from build123d import *

# Parameters (mm, degrees)
SKETCH1_W                 = 127
SKETCH1_H                 = 127
BOSS_EXTRUDE1_DEPTH       = 3.175
SKETCH2_W                 = 3.175
SKETCH2_H                 = 25.4
CUT_EXTRUDE1_DEPTH        = 6.35
LPATTERN1_COUNT           = 3
LPATTERN1_PITCH           = 50.8
LPATTERN1_COUNT_DIR2      = 2
LPATTERN1_PITCH_DIR2      = 123.825
SKETCH3_W                 = 25.4
SKETCH3_H                 = 3.175
CUT_EXTRUDE2_DEPTH        = 6.35
LPATTERN2_COUNT           = 3
LPATTERN2_PITCH           = 50.8
LPATTERN2_COUNT_DIR2      = 2
LPATTERN2_PITCH_DIR2      = 123.825
SKETCH4_W                 = 17.145
SKETCH4_H                 = 4.3942
SKETCH4_W_2               = 3.302
SKETCH4_H_2               = 8.89
CUT_EXTRUDE3_DEPTH        = 8.89
SKETCH5_W                 = 4.3942
SKETCH5_H                 = 17.145
SKETCH5_W_2               = 8.89
SKETCH5_H_2               = 3.302
CUT_EXTRUDE4_DEPTH        = 30.48
LPATTERN3_COUNT           = 2
LPATTERN3_PITCH           = 50.8
MIRROR2_COPY_1_SKETCH_W   = 4.3942
MIRROR2_COPY_1_SKETCH_H   = 17.145
MIRROR2_COPY_1_SKETCH_W_2 = 8.89
MIRROR2_COPY_1_SKETCH_H_2 = 3.302
MIRROR2_COPY_1_DEPTH      = 30.48
F_4_CLEARANCE_HOLE3_D     = 3.2639
F_4_CLEARANCE_HOLE3_DEPTH = 10.16
F_4_CLEARANCE_HOLE3_TIP   = 0.980574487
F_4_CLEARANCE_HOLE4_D     = 3.2639
F_4_CLEARANCE_HOLE4_DEPTH = 10.16
F_4_CLEARANCE_HOLE4_TIP   = 0.980574487


with BuildPart() as part:
    # Sketch1 → Boss-Extrude1 (new body)
    with BuildSketch(Plane(origin=(0, 0, 0), x_dir=(1, 0, 0), z_dir=(0, 1, 0))):
        with Locations((63.5, 63.5)):
            Rectangle(SKETCH1_W, SKETCH1_H)
    extrude(amount=BOSS_EXTRUDE1_DEPTH)

    # Sketch2 → Cut-Extrude1 (cut)
    with BuildSketch(Plane(origin=(0, 3.175, 0), x_dir=(1, 0, 0), z_dir=(0, 1, 0))):
        with Locations((1.5875, 114.3)):
            Rectangle(SKETCH2_W, SKETCH2_H)
    cut_extrude1 = extrude(amount=-CUT_EXTRUDE1_DEPTH, mode=Mode.SUBTRACT)

    # LPattern1: Cut-Extrude1 3 × 2
    with Locations(*[(j * LPATTERN1_PITCH_DIR2, 0, i * LPATTERN1_PITCH) for i in range(LPATTERN1_COUNT) for j in range(LPATTERN1_COUNT_DIR2) if (i, j) != (0, 0)]):
        add(cut_extrude1, mode=Mode.SUBTRACT)

    # Sketch3 → Cut-Extrude2 (cut)
    with BuildSketch(Plane(origin=(0, 3.175, 0), x_dir=(1, 0, 0), z_dir=(0, 1, 0))):
        with Locations((38.1, 1.5875)):
            Rectangle(SKETCH3_W, SKETCH3_H)
    cut_extrude2 = extrude(amount=-CUT_EXTRUDE2_DEPTH, mode=Mode.SUBTRACT)

    # LPattern2: Cut-Extrude2 3 × 2
    with Locations(*[(i * LPATTERN2_PITCH, 0, -j * LPATTERN2_PITCH_DIR2) for i in range(LPATTERN2_COUNT) for j in range(LPATTERN2_COUNT_DIR2) if (i, j) != (0, 0)]):
        add(cut_extrude2, mode=Mode.SUBTRACT)

    # Sketch4 → Cut-Extrude3 (cut)
    with BuildSketch(Plane(origin=(0, 3.175, 0), x_dir=(1, 0, 0), z_dir=(0, 1, 0))):
        with Locations((115.2525, 63.5)):
            Rectangle(SKETCH4_W, SKETCH4_H)
        with Locations((117.475, 63.5)):
            Rectangle(SKETCH4_W_2, SKETCH4_H_2)
    cut_extrude3 = extrude(amount=-CUT_EXTRUDE3_DEPTH, mode=Mode.SUBTRACT)

    # Sketch5 → Cut-Extrude4 (cut)
    with BuildSketch(Plane(origin=(0, 3.175, 0), x_dir=(1, 0, 0), z_dir=(0, 1, 0))):
        with Locations((38.1, 11.7475)):
            Rectangle(SKETCH5_W, SKETCH5_H)
        with Locations((38.1, 9.525)):
            Rectangle(SKETCH5_W_2, SKETCH5_H_2)
    cut_extrude4 = extrude(amount=-CUT_EXTRUDE4_DEPTH, mode=Mode.SUBTRACT)

    # LPattern3: Cut-Extrude4 ×2
    with Locations(*[(i * LPATTERN3_PITCH, 0, 0) for i in range(1, LPATTERN3_COUNT)]):
        add(cut_extrude4, mode=Mode.SUBTRACT)

    # Mirror2: Cut-Extrude4 across plane
    add(cut_extrude4.mirror(Plane.XY.offset(-63.5)), mode=Mode.SUBTRACT)

    # Mirror2 copy 1 sketch → Mirror2 copy 1 (cut)
    with BuildSketch(Plane(origin=(50.8, 3.175, -127), x_dir=(1, 0, 0), z_dir=(0, 1, 0))):
        with Locations((38.1, -11.7475)):
            Rectangle(MIRROR2_COPY_1_SKETCH_W, MIRROR2_COPY_1_SKETCH_H)
        with Locations((38.1, -9.525)):
            Rectangle(MIRROR2_COPY_1_SKETCH_W_2, MIRROR2_COPY_1_SKETCH_H_2)
    extrude(amount=-MIRROR2_COPY_1_DEPTH, mode=Mode.SUBTRACT)

    # #4 Clearance Hole3
    with Locations(Plane(origin=(0, 3.175, 0), x_dir=(1, 0, 0), z_dir=(0, 1, 0))):
        with Locations((21.082, 82.931), (48.26, 82.931), (48.26, 40.513)):
            Hole(F_4_CLEARANCE_HOLE3_D / 2, depth=F_4_CLEARANCE_HOLE3_DEPTH)
            with Locations((0, 0, -(F_4_CLEARANCE_HOLE3_DEPTH + F_4_CLEARANCE_HOLE3_TIP / 2))):  # 118° drill point
                Cone(0, F_4_CLEARANCE_HOLE3_D / 2, F_4_CLEARANCE_HOLE3_TIP, mode=Mode.SUBTRACT)

    # #4 Clearance Hole4
    with Locations(Plane(origin=(0, 3.175, 0), x_dir=(1, 0, 0), z_dir=(0, 1, 0))):
        with Locations((63.5, 19.05)):
            Hole(F_4_CLEARANCE_HOLE4_D / 2, depth=F_4_CLEARANCE_HOLE4_DEPTH)
            with Locations((0, 0, -(F_4_CLEARANCE_HOLE4_DEPTH + F_4_CLEARANCE_HOLE4_TIP / 2))):  # 118° drill point
                Cone(0, F_4_CLEARANCE_HOLE4_D / 2, F_4_CLEARANCE_HOLE4_TIP, mode=Mode.SUBTRACT)

    # Mirror3: Cut-Extrude3 across plane
    add(cut_extrude3.mirror(Plane.ZY.offset(-63.5)), mode=Mode.SUBTRACT)


solid = part.part
Work out the finished part from the listing and answer in its coordinate system (mm). A direction names the side the tool comes from. Give positions to 0.01 mm unless a question says otherwise; leave off trailing zeros. Order: outer loops, then holes, each group sorted by start corner. A loop starts at its lowest first (then second) coordinate and runs counter-clockwise, first axis right, second up. Notation, with made-up numbers: (-39.5, 45.5) -> (-33.5, 45.5) arc R15 cw to (-33.5, 61.5) -> close; hole circle Ø2 at (72, 49.5). An arc over 180 degrees is marked (long way). One line per item, written item: value.
Item 1: Find section B-B, the plane x = 48.26. Give the vertices of the cut face in (y, z) (3 decimals).
Answer sheet:
outline: (0, -123.825) -> (3.175, -123.825) -> (3.175, -84.563) -> (0, -84.563) -> close; (0, -81.299) -> (3.175, -81.299) -> (3.175, -42.145) -> (0, -42.145) -> close; (0, -38.881) -> (3.175, -38.881) -> (3.175, -3.175) -> (0, -3.175) -> close
Item 2: Determine the mould class of faces 1 (the flat face through (76.2, 2, -2)), 2 (the flat face through (121, 2, -65.697)), 3 (the flat face through (42.545, 2, -10)), 4 (the flat face through (123.825, 2, -114)) for opening direction X: released by +X, released by -X, zero draft, split by the parting line, or undercut.
Answer sheet:
face 1: undercut
face 2: zero draft
face 3: undercut
face 4: released by +X
Item 3: A tool of negligible diameter and unlimited length cuts with its end or side. For faces 5 (the flat face through (117, 2, -67.945)), 6 (the flat face through (40.297, 2, -5)), 7 (the flat face through (91.097, 2, -111)), 8 (the flat face through (125, 2, -101.6)), from which of +Z, -Z, +X, -X, +Y, -Y can it reach the whole face along a straight path? Write none if from no direction.
Answer sheet:
face 5: +Y, -Y
face 6: +Z, +Y, -Y
face 7: -Z, +Y, -Y
face 8: -Z, +X, +Y, -Y
Item 4: Find section C-C, the plane y = 1.7. State how many separate pieces and enclosed holes the cut face has, plus the area to 3 significant figures.
Answer sheet:
separate pieces: 1
enclosed holes: 4
area: 14,700 mm²
Item 5: Find section A-A, the plane x = 63.5. Give the vertices of the cut face in (y, z) (3 decimals).
Answer sheet:
outline: (0, -127) -> (3.175, -127) -> (3.175, -20.682) -> (0, -20.682) -> close; (0, -17.418) -> (3.175, -17.418) -> (3.175, 0) -> (0, 0) -> close
Item 6: Flat-ended cylindrical pins translate along their axes: P1, Ø4, axis at x = 63.5, z = -19.05, coming from the +Y side (3 decimals); P2, Ø1.8, axis at x = 41, y = 2, coming from the -Z side (3 decimals); P3, Ø1, axis at x = 125, y = 1, coming from the +Z side; P4, Ø1.1, axis at x = 41, y = 2, coming from the +Z side (3 decimals). Find the tip coordinate at first contact, or state that the pin passes through.
Answer sheet:
P1: y = 3.175
P2: z = -123.825
P3: z = -25.4
P4: z = -3.175
Item 7: Straight lines are drawn through the part: probe 1 along X at (y, z) = (2.7, -5.5) (3 decimals); probe 2 along Z at (x, y) = (48.26, 2.5) (3 decimals); probe 3 along X at (y, z) = (2.25, -19.05) (3 decimals). For each, find the intervals that lie inside material, in ascending order.
Answer sheet:
probe 1: 3.175 to 35.903, 40.297 to 86.703, 91.097 to 123.825
probe 2: -123.825 to -84.563, -81.299 to -42.145, -38.881 to -3.175
probe 3: 3.175 to 35.903, 40.297 to 61.868, 65.132 to 86.703, 91.097 to 123.825
Item 8: Find section D-D, the plane x = 98. Give the vertices of the cut face in (y, z) (3 decimals), plus the area to 3 significant figures.
Answer sheet:
outline: (0, -123.825) -> (3.175, -123.825) -> (3.175, -3.175) -> (0, -3.175) -> close
area: 383 mm²
